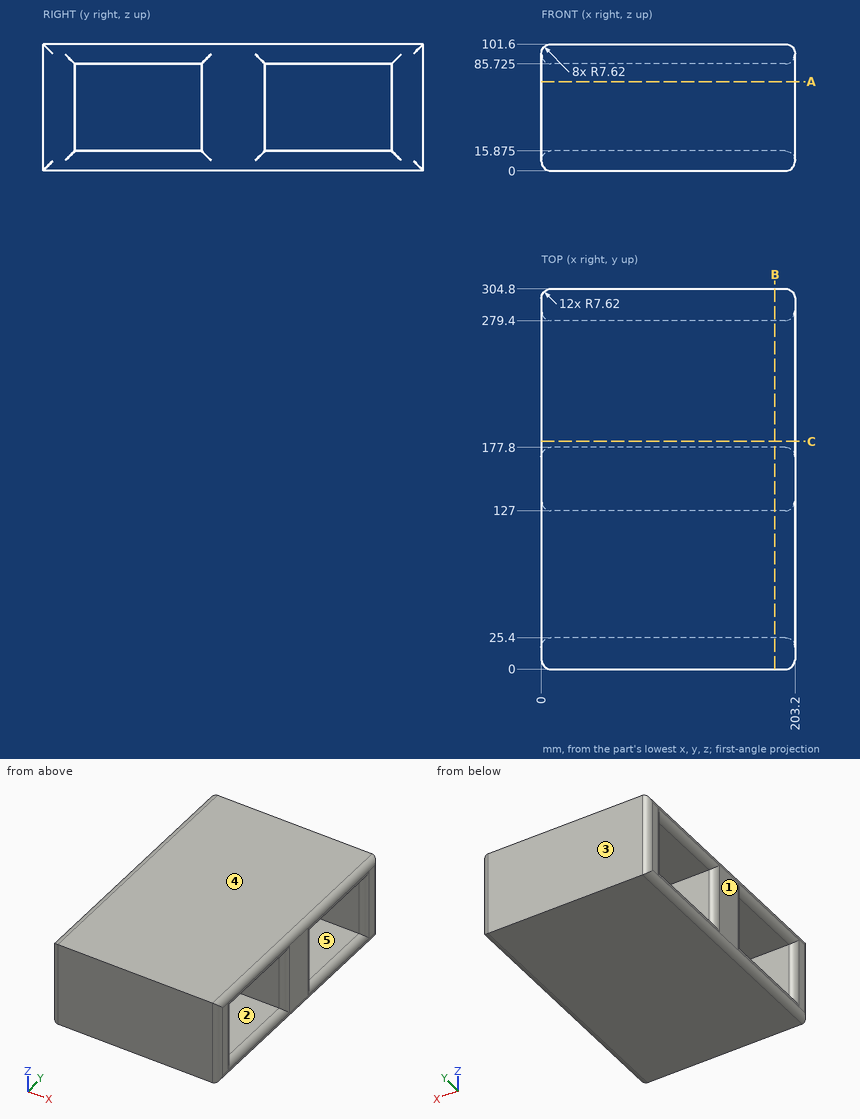
The drawing under review shows one solid part. Ordinate dimensions are in mm from its lowest x, y, z. A direction names the side the tool comes from. Round coordinates to 2 decimals unless told otherwise and drop trailing zeros. Order: outer loops, then holes, each group sorted by start corner. A loop starts at its lowest first (then second) coordinate and runs counter-clockwise, first axis right, second up. Notation, with made-up numbers: (54, 45.25) -> (64, 45.25) arc R14 cw to (64, 51.25) -> close; hole circle Ø11 at (47.5, 61). An arc over 180 degrees is marked (long way). Use a Markdown table: item, result.
Q1. Mouldability with a two-part tool opening along Y and no side actions: class the marked faces 3, 4 and 5 as +Y half, -Y half, draft (parallel to the pull), parting line (faces both ways), or undercut.
Values:
| item | result |
|---|---|
| face 3 | +Y half |
| face 4 | draft |
| face 5 | undercut |
Q2. Tool access review of the marked faces 1 and 2: name each direction out of +Z, -Z, +X, -X, +Y, -Y from which nothing blocks a thin tool from reaching the whole face with its end or side.
Values:
| item | result |
|---|---|
| face 1 | +Z, -Z, -X, +Y, -Y |
| face 2 | +X, -X |
Q3. We need section B-B on x = 187. Write out the cut boundary in (y, z) (3 decimals).
Values:
| item | result |
|---|---|
| outline | (0, 0) -> (304.8, 0) -> (304.8, 101.6) -> (0, 101.6) -> close; hole (25.4, 15.875) -> (127, 15.875) -> (127, 85.725) -> (25.4, 85.725) -> close; hole (177.8, 15.875) -> (279.4, 15.875) -> (279.4, 85.725) -> (177.8, 85.725) -> close |
Q4. For line 1 (Y direction, x = 60.5, z = 54); line 2 (Z direction, x = 84.5, y = 90.5) (3 decimals); line 3 (X direction, y = 18, z = 38.5), list the stretches that pass through material, from the lowest coordinate up.
Values:
| item | result |
|---|---|
| line 1 | y = 0 to 25.4, 127 to 177.8, 279.4 to 304.8 |
| line 2 | z = 0 to 15.875, 85.725 to 101.6 |
| line 3 | x = 0 to 203.2 |
Q5. Clearance check with a flat-ended pin moving along its axis: P1, Ø5, axis at y = 177, z = 77, coming from the +X side. State where the tip first meets the part, or that it passes through.
Values:
| item | result |
|---|---|
| P1 | stops at x = 201.86 |
Q6. We need section C-C on y = 182.5. Write out the cut boundary in (x, z) (3 decimals), then the cut area to 3 significant figures.
Values:
| item | result |
|---|---|
| outline | (0, 7.62) arc R7.62 ccw to (7.62, 0) -> (195.58, 0) arc R7.62 ccw to (203.2, 7.62) -> (203.2, 8.255) arc R7.62 ccw to (195.58, 15.875) -> (7.62, 15.875) arc R7.62 ccw to (0, 8.255) -> close; (0, 93.345) arc R7.62 ccw to (7.62, 85.725) -> (195.58, 85.725) arc R7.62 ccw to (203.2, 93.345) -> (203.2, 93.98) arc R7.62 ccw to (195.58, 101.6) -> (7.62, 101.6) arc R7.62 ccw to (0, 93.98) -> close |
| area | 6,350 mm^2 |
Q7. We need section A-A on z = 71.5. Write out the cut boundary in (x, y), then the cut area to 3 significant figures.
Values:
| item | result |
|---|---|
| outline | (0, 7.62) arc R7.62 ccw to (7.62, 0) -> (195.58, 0) arc R7.62 ccw to (203.2, 7.62) -> (203.2, 17.78) arc R7.62 ccw to (195.58, 25.4) -> (7.62, 25.4) arc R7.62 ccw to (0, 17.78) -> close; (0, 134.62) arc R7.62 ccw to (7.62, 127) -> (195.58, 127) arc R7.62 ccw to (203.2, 134.62) -> (203.2, 170.18) arc R7.62 ccw to (195.58, 177.8) -> (7.62, 177.8) arc R7.62 ccw to (0, 170.18) -> close; (0, 287.02) arc R7.62 ccw to (7.62, 279.4) -> (195.58, 279.4) arc R7.62 ccw to (203.2, 287.02) -> (203.2, 297.18) arc R7.62 ccw to (195.58, 304.8) -> (7.62, 304.8) arc R7.62 ccw to (0, 297.18) -> close |
| area | 20,500 mm^2 |
